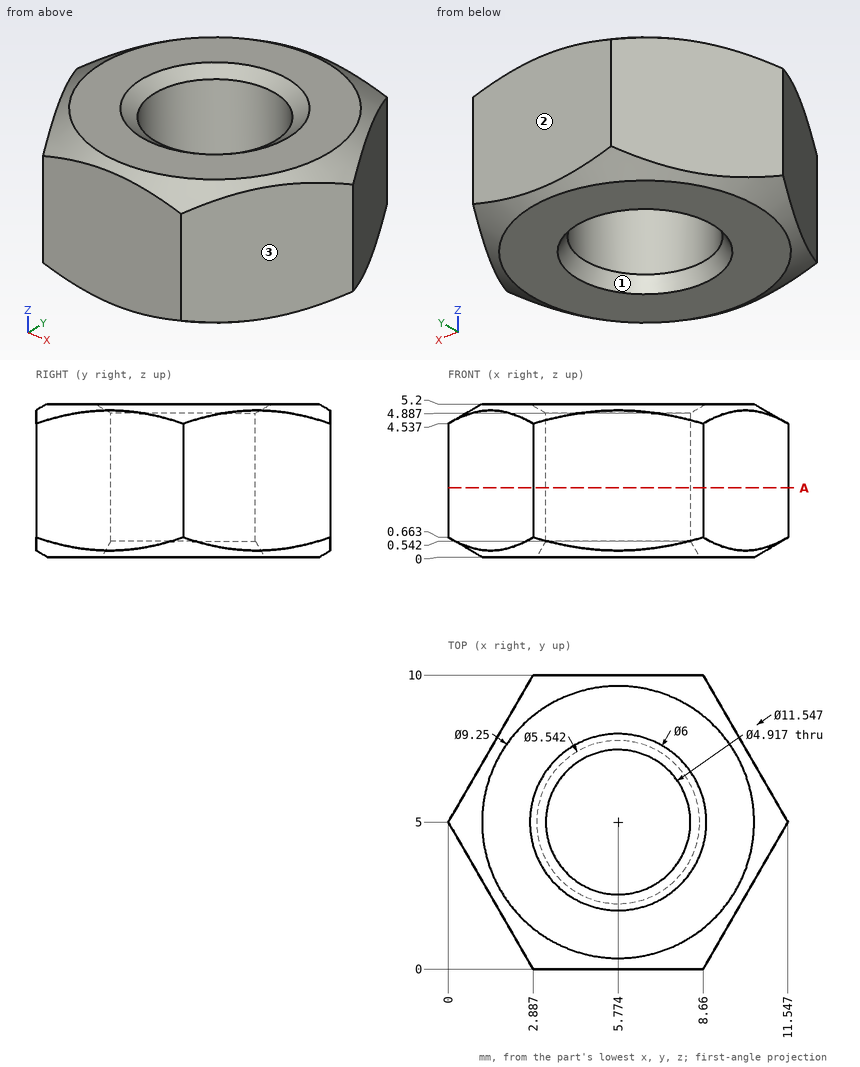
For this review, use the dimensioned drawing (mm, ordinates from the lowest corner) and the shaded views. Give positions to 0.01 mm unless a question says otherwise; leave off trailing zeros. Order: outer loops, then holes, each group sorted by start corner. A loop starts at its lowest first (then second) coordinate and runs counter-clockwise, first axis right, second up. Notation, with made-up numbers: M 77.5,-32 L 127.5,-32 A17 cw 127.5,-9 Z; hole C 18.25,45.25 d11. An arc over 180 degrees is marked long. Use one line per item in the form item = value. Start each with the question number.
Item 1: The part is to be moulded in two halves that separate along X. For the marked faces 1, 2 and 3, say which applies: pulls with the +X half, pulls with the -X half, needs draft (parallel to the pull), parting line crosses it, or undercut.
Item 2: We need section A-A on z = 2.35. Give the boundary of the cut face in (x, y).
Item 3: Insertion check: pin 1 Ø1.5 at (y, z) = (7.5, 1.5) entering from -X; pin 2 Ø2 at (y, z) = (2, 2.5) entering from -X (1 decimal); pin 3 Ø1.5 at (x, z) = (1.5, 4) entering from -Y (1 decimal). Each pin has a flat end and moves straight along its axis. Give the tip position at first contact, or say it passes through.
Item 4: To check wall thickness, follow line 1 along X through (y, z) = (6, 3.35); line 2 along Y through (x, z) = (4.5, 4.55) (1 decimal); line 3 along X through (y, z) = (7, 1.7) (1 decimal). State the ranges of each line that lie inside material, in increasing order. Write a range as from..to.
Completed:
q1.face_1 = undercut
q1.face_2 = needs draft
q1.face_3 = pulls with the +X half
q2.outline = M 0,5 L 2.89,0 L 8.66,0 L 11.55,5 L 8.66,10 L 2.89,10 Z; hole C 5.77,5 d4.92
q3.pin_1 = 1.01
q3.pin_2 = 1.2
q3.pin_3 = 1.1
q4.line_1 = 0.58..3.53, 8.02..10.97
q4.line_2 = 0..2.9, 7.1..10
q4.line_3 = 1.2..4.3, 7.2..10.4
